Geometry: see drawing. Coordinates: mm, zero at the bounding-box minimum. A direction names the side the tool comes from. Give positions to 0.01 mm unless a question says otherwise; leave off trailing zeros. Loops run counter-clockwise (first coordinate to the right, second up) from the corner with the lowest first, then second, coordinate; pieces in that order, holes last. Notation, with made-up numbers: M 49,25.25 L 91,25.25 A19 ccw 91,42.25 Z; hole C 35.5,-24 d10. An arc over 180 degrees is marked long. Put each result on its own line as item: value.
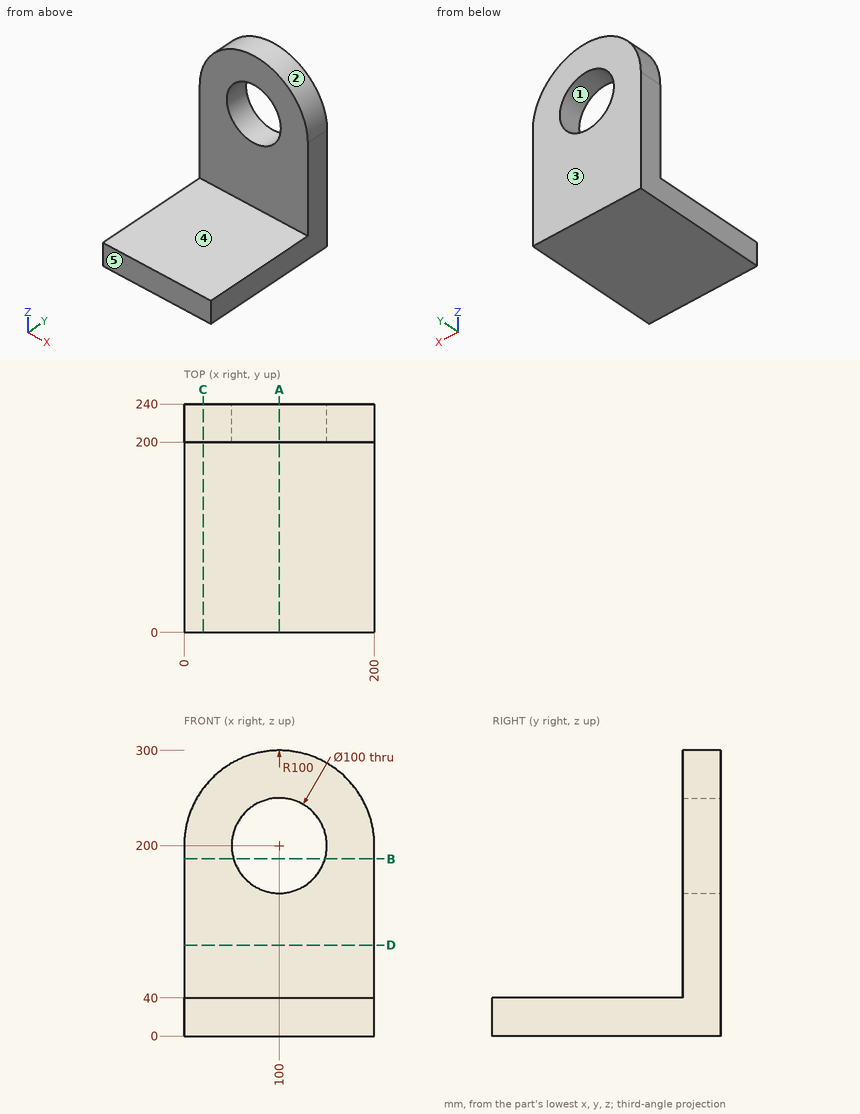
Item 1: Section C-C on x = 20. Output: boundary loops of the cut face in (y, z), then the cut area to 3 significant figures.
Output values:
outline: M 0,0 L 240,0 L 240,260 L 200,260 L 200,40 L 0,40 Z
area: 18,400 mm²
Item 2: Section D-D on z = 95.5. Output: boundary loops of the cut face in (x, y).
Output values:
outline: M 0,200 L 200,200 L 200,240 L 0,240 Z
Item 3: Section B-B on z = 186. Output: boundary loops of the cut face in (x, y), then the cut area to 3 significant figures.
Output values:
outline: M 0,200 L 52,200 L 52,240 L 0,240 Z; M 148,200 L 200,200 L 200,240 L 148,240 Z
area: 4,160 mm²
Item 4: Set-up query: the marked faces 4 and 5. Return all of +Z, -Z, +X, -X, +Y, -Y with unobstructed straight access to the full face (end or side cutting, diameter ignored); none if empty.
Output values:
face 4: +Z, +X, -X, -Y
face 5: +Z, -Z, +X, -X, -Y
Item 5: Pin query (flat end, axial travel): pin 1 Ø4 at (x, y) = (159, 99) entering from +Z. Return the tip coordinate at first contact, or that it passes through.
Output values:
pin 1: z = 40
Item 6: Mould query, pull axis Z, two halves, no side actions, for the marked faces 1, 2 and 3. Classes: pulls with the +Z half, pulls with the -Z half, needs draft (parallel to the pull), parting line crosses it, or undercut.
Output values:
face 1: undercut
face 2: pulls with the +Z half
face 3: needs draft
Item 7: Line query: probe 1 along Z at (x, y) = (100, 227); probe 2 along Y at (x, z) = (161, 64); probe 3 along Z at (x, y) = (33, 120). Output: solid intervals per line, ascending. Write a range as [from, to].
Output values:
probe 1: [0, 150], [250, 300]
probe 2: [200, 240]
probe 3: [0, 40]
Item 8: Section A-A on x = 100. Output: boundary loops of the cut face in (y, z), then the cut area to 3 significant figures.
Output values:
outline: M 0,0 L 240,0 L 240,150 L 200,150 L 200,40 L 0,40 Z; M 200,250 L 240,250 L 240,300 L 200,300 Z
area: 16,000 mm²
